Geometry: final body of the model. Coordinates: model frame, mm. Face numbers are marked on the shaded views. A direction names the side the tool comes from. Give positions to 0.01 mm unless a question says otherwise; leave off trailing zeros. Loops run counter-clockwise (first coordinate to the right, second up) from the corner with the lowest first, then second, coordinate; pieces in that order, holes last.
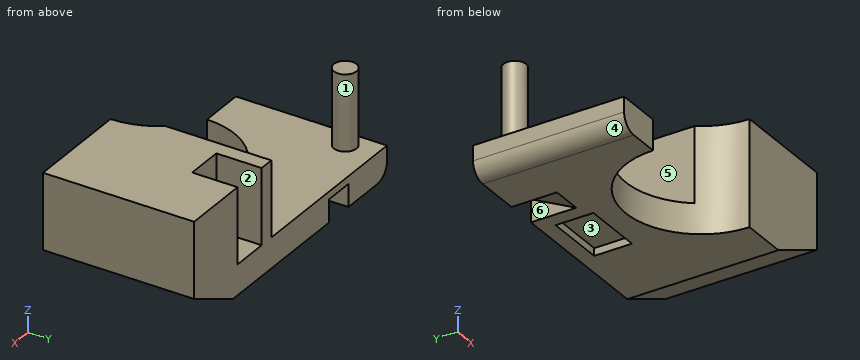
```python
from build123d import *

# Parameters (mm, degrees)
SKICA1_W                 = 200
SKICA1_H                 = 100
P_IDAT_VYSUNUT_M1_DEPTH  = 20
P_IDAT_VYSUNUT_M2_DEPTH  = 50
ODEBRAT_VYSUNUT_M1_REACH = 236.307
SKICA4_R                 = 50
SKICA7_R                 = 7.5
P_IDAT_VYSUNUT_M3_DEPTH  = 50
ODEBRAT_VYSUNUT_M3_DEPTH = 10
ZAOBLIT1_R               = 10
ZKOSEN_1_SIZE            = 40
ZKOSEN_1_SIZE2           = 20
SKICA9_W                 = 40
SKICA9_H                 = 25
ODEBRAT_VYSUNUT_M4_DEPTH = 5


with BuildPart() as part:
    # Skica1 → Přidat vysunutím1 (new body)
    with BuildSketch(Plane.XY):
        with Locations((100, 50)):
            Rectangle(SKICA1_W, SKICA1_H)
    extrude(amount=P_IDAT_VYSUNUT_M1_DEPTH)

    # Skica2 → Přidat vysunutím2 (add)
    with BuildSketch(Plane.XY.offset(20)):
        Polygon((120, 0), (200, 0), (200, 100), (155, 100), (155, 70), (130, 70), (130, 100), (120, 100), align=None)
    extrude(amount=P_IDAT_VYSUNUT_M2_DEPTH)

    # Odebrat vysunutím1: up to this face of the body (flat: up to its plane)
    odebrat_vysunut_m1_end = Plane(part.part.faces().sort_by_distance((161.810344828, 46.379310345, 70))[0])
    # Skica4 → Odebrat vysunutím1 (cut, up to the picked face)
    with BuildSketch(Plane(origin=(0, 0, 0), x_dir=(-1, 0, 0), z_dir=(0, 0, -1)), mode=Mode.PRIVATE) as odebrat_vysunut_m1_sk1:
        with Locations((-80, 0)):
            Circle(SKICA4_R)
    odebrat_vysunut_m1_tool1 = split(extrude(odebrat_vysunut_m1_sk1.sketch, amount=-ODEBRAT_VYSUNUT_M1_REACH, mode=Mode.PRIVATE), bisect_by=odebrat_vysunut_m1_end, keep=Keep.BOTH, mode=Mode.PRIVATE)
    add(odebrat_vysunut_m1_tool1.solids().sort_by(Axis((80, 0, 0), (0, 0, 1)))[0], mode=Mode.SUBTRACT)

    # Skica7 → Přidat vysunutím3 (add)
    with BuildSketch(Plane.XY.offset(20)):
        with Locations(Location((12, 80, 0), (0, 0, 180))):
            Circle(SKICA7_R)
    extrude(amount=P_IDAT_VYSUNUT_M3_DEPTH)

    # Skica8 → Odebrat vysunutím3 (cut, symmetric)
    with BuildSketch(Plane.ZY.offset(-50)):
        Polygon((0, 100), (0, 70), (15, 100), align=None)
    extrude(amount=ODEBRAT_VYSUNUT_M3_DEPTH, both=True, mode=Mode.SUBTRACT)

    # Zaoblit1
    zaoblit1_edges = [part.edges().sort_by_distance(p)[0] for p in [
        (0, 50, 0),
    ]]
    fillet(zaoblit1_edges, radius=ZAOBLIT1_R)

    # Zkosení1
    zkosen_1_edges = [part.edges().sort_by_distance(p)[0] for p in [
        (200, 50, 0),
    ]]
    zkosen_1_side = [part.faces().sort_by_distance(p)[0] for p in [
        (114.06340684, 56.357779944, 0),
    ]]
    chamfer(zkosen_1_edges, length=ZKOSEN_1_SIZE, length2=ZKOSEN_1_SIZE2, reference=zkosen_1_side[0])

    # Skica9 → Odebrat vysunutím4 (cut)
    with BuildSketch(Plane(origin=(0, 0, 0), x_dir=(-1, 0, 0), z_dir=(0, 0, -1))):
        with Locations((-90, 77.5)):
            Rectangle(SKICA9_W, SKICA9_H)
    extrude(amount=-ODEBRAT_VYSUNUT_M4_DEPTH, mode=Mode.SUBTRACT)


solid = part.part
```
Q1. Material intervals for probe 1 along X at (y, z) = (94.5, 27); probe 2 along X at (y, z) = (31, 47); probe 3 along Z at (x, y) = (20, 65.5), sorted ascending.
Q2. Pin query (flat end, axial travel): pin 1 Ø1.5 at (y, z) = (72, 2.5) entering from +X; pin 2 Ø10 at (y, z) = (30, 40.5) entering from -X; pin 3 Ø2.5 at (x, z) = (91, 2) entering from -Y. Return the tip coordinate at first contact, or that it passes through.
Q3. Section query B-B, the plane y = 80. Return loops of the section in (x, z).
Q4. Section query A-A, the plane z = 65. Return loops of the section in (x, y), and give its area (3 significant figures).
Q5. Mould query, pull axis Y, two halves, no side actions, for the marked faces 1, 2 and 3. Classes: +Y half, -Y half, draft (parallel to the pull), parting line (faces both ways), or undercut.
Q6. Section query C-C, the plane x = 12. Return loops of the section in (y, z), and give its area (3 significant figures).
Q7. Reachability of the marked faces 4, 5 and 6 from +Z, -Z, +X, -X, +Y, -Y: full face, straight path, thin tool, end or side. Return the list, or none.
Q8. Section query D-D, the plane y = 17.5. Return loops of the section in (x, z), and give its area (3 significant figures).
Resolved:
1. probe 1: x = 120 to 130, 155 to 200
1. probe 2: x = 120 to 200
1. probe 3: z = 0 to 20
2. pin 1: stops at x = 166.5
2. pin 2: stops at x = 120
2. pin 3: stops at y = 48.48
3. outline: (0, 10) arc R10 ccw to (10, 0) - (40, 0) - (40, 5) - (60, 5) - (60, 0) - (70, 0) - (70, 5) - (110, 5) - (110, 0) - (160, 0) - (200, 20) - (200, 70) - (155, 70) - (155, 20) - (130, 20) - (130, 70) - (120, 70) - (120, 20) - (19.5, 20) - (19.5, 70) - (4.5, 70) - (4.5, 20) - (0, 20) - close
4. outline: circle Ø15 at (12, 80); (120, 30) arc R50 cw to (130, 0) - (200, 0) - (200, 100) - (155, 100) - (155, 70) - (130, 70) - (130, 100) - (120, 100) - close
4. area: 7,220 mm2
5. face 1: parting line
5. face 2: draft
5. face 3: undercut
6. outline: (0, 0) - (100, 0) - (100, 20) - (87.5, 20) - (87.5, 70) - (72.5, 70) - (72.5, 20) - (0, 20) - close
6. area: 2,750 mm2
7. face 4: -Z, -X, +Y, -Y
7. face 5: +Z, +Y, -Y
7. face 6: -Z, +Y
8. outline: (0, 10) arc R10 ccw to (10, 0) - (33.16, 0) - (33.16, 20) - (0, 20) - close; (126.84, 0) - (160, 0) - (200, 20) - (200, 70) - (126.84, 70) - close
8. area: 5,360 mm2
